Design review of the part built by this model. Coordinates are the model's own, in mm. A direction names the side the tool comes from. Coordinates: 2 decimals unless noted, no trailing zeros. Loops run counter-clockwise (first coordinate to the right, second up) from the corner with the lowest first, then second, coordinate; pieces in that order, holes last. Notation, with made-up numbers: (61, 11.25) - (113, 11.25) arc R15 ccw to (113, 23.25) - close; hole circle Ø11 at (-27, 79). An arc over 180 degrees is marked (long way). One line per question, with ' | ' between items.
from build123d import *

# Parameters (mm, degrees)
PAD_DEPTH       = 3.4
FILLET_R        = 4
SKETCH001_R     = 18
SKETCH001_R_2   = 6.25
PAD001_DEPTH    = 36
SKETCH002_W     = 12
SKETCH002_H     = 42
SKETCH002_R     = 2.65
PAD002_DEPTH    = 48
FILLET002_R     = 2
SKETCH004_W     = 8
SKETCH004_H     = 36.680408
PAD010_DEPTH    = 68
CHAMFER_SIZE    = 20
CHAMFER001_SIZE = 2
SKETCH005_R     = 1.5
POCKET_DEPTH    = 10


with BuildPart() as part:
    # Sketch → Pad (new body)
    with BuildSketch(Plane.XY):
        with BuildLine():
            Line((-65, 0), (-65, -60))
            Line((-65, -60), (65, -60))
            Line((65, -60), (65, 0))
            ThreePointArc((65, 0), (0, 45.409517), (-65, 0))
        make_face()
    extrude(amount=PAD_DEPTH)

    # Fillet
    fillet_edges = [part.edges().sort_by_distance(p)[0] for p in [
        (65, -60, 1.7),
        (-65, -60, 1.7),
    ]]
    fillet(fillet_edges, radius=FILLET_R)

    # Sketch001 (on Face6 of Pad) → Pad001 (join)
    with BuildSketch(Plane.XY.offset(3.4)):
        with Locations((42, -6)):
            Circle(SKETCH001_R)
        with Locations((42, -6)):
            Circle(SKETCH001_R_2, mode=Mode.SUBTRACT)
    pad001 = extrude(amount=PAD001_DEPTH)

    # Mirrored: Pad001 across YZ
    add(pad001.mirror(Plane.YZ))

    # Sketch002 (on Face5 of Mirrored) → Pad002 (join)
    with BuildSketch(Plane.XY.offset(3.4)):
        with Locations((-27.4, -35)):
            Rectangle(SKETCH002_W, SKETCH002_H)
        with Locations((-27.4, -26)):
            Circle(SKETCH002_R, mode=Mode.SUBTRACT)
        with Locations((-27.4, -44)):
            Circle(SKETCH002_R, mode=Mode.SUBTRACT)
    pad002 = extrude(amount=PAD002_DEPTH)

    # Mirrored001: Pad002 across Sketch002 V_Axis
    add(pad002.mirror(Plane(origin=(0, 0, 3.4), x_dir=(0, 0, 1), z_dir=(1, 0, 0))))

    # Fillet002
    fillet002_edges = [part.edges().sort_by_distance(p)[0] for p in [
        (33.4, -14, 45.4),
        (-33.4, -14, 45.4),
    ]]
    fillet(fillet002_edges, radius=FILLET002_R)

    # Sketch004 (on Face6 of Fillet002) → Pad010 (join)
    with BuildSketch(Plane.XY.offset(3.4)):
        with Locations((37.4, -37.659796)):
            Rectangle(SKETCH004_W, SKETCH004_H)
    extrude(amount=PAD010_DEPTH)

    # Chamfer
    chamfer_edges = [part.edges().sort_by_distance(p)[0] for p in [
        (37.4, -56, 71.4),
    ]]
    chamfer(chamfer_edges, length=CHAMFER_SIZE)

    # Chamfer001
    chamfer001_edges = [part.edges().sort_by_distance(p)[0] for p in [
        (33.4, -46, 61.4),
        (33.4, -27.659796, 71.4),
    ]]
    chamfer(chamfer001_edges, length=CHAMFER001_SIZE)

    # Sketch005 (on Face4 of Chamfer001) → Pocket (cut)
    with BuildSketch(Plane.YZ.offset(41.4)):
        with Locations((-32.7462, 64.451439)):
            Circle(SKETCH005_R)
        with Locations((-22.2462, 64.451439)):
            Circle(SKETCH005_R)
    extrude(amount=-POCKET_DEPTH, mode=Mode.SUBTRACT)


solid = part.part
Q1. Take a section at A-A (z = 13). Give the boundary of the cut face in (x, y), plus the area to 3 significant figures.
Returned:
outline: (-33.4, -56) - (-21.4, -56) - (-21.4, -14) - (-25.88, -14) arc R18 ccw (long way) to (-33.4, -21.81) - close; (21.4, -56) - (41.4, -56) - (41.4, -23.99) arc R18 ccw (long way) to (25.88, -14) - (21.4, -14) - close; hole circle Ø12.5 at (-42, -6); hole circle Ø5.3 at (-27.4, -44); hole circle Ø5.3 at (-27.4, -26); hole circle Ø5.3 at (27.4, -44); hole circle Ø5.3 at (27.4, -26); hole circle Ø12.5 at (42, -6) | area: 2,900 mm²
Q2. Take a section at C-C (x = 27.4). Give the boundary of the cut face in (y, z), plus the area to 3 significant figures.
Returned:
outline: (-60, 0) - (39.76, 0) - (39.76, 3.4) - (4.53, 3.4) - (4.53, 39.4) - (-14, 39.4) - (-14, 51.4) - (-23.35, 51.4) - (-23.35, 3.4) - (-28.65, 3.4) - (-28.65, 51.4) - (-41.35, 51.4) - (-41.35, 3.4) - (-46.65, 3.4) - (-46.65, 51.4) - (-56, 51.4) - (-56, 3.4) - (-60, 3.4) - close | area: 2,510 mm²
Q3. To check wall thickness, follow line 1 along Y through (x, z) = (-26.5, 7.5); line 2 along Y through (x, z) = (-42, 27); line 3 along X through (y, z) = (-32, 9.5). State the ranges of each line that lie inside material, in increasing order.
Returned:
line 1: y = -56 to -46.49, -41.51 to -28.49, -23.51 to 3.15 | line 2: y = -24 to -12.25, 0.25 to 12 | line 3: x = -33.4 to -21.4, 21.4 to 41.4
Q4. Take a section at D-D (y = -38). Give the boundary of the cut face in (x, z).
Returned:
outline: (-65, 0) - (65, 0) - (65, 3.4) - (41.4, 3.4) - (41.4, 69.4) - (35.4, 69.4) - (33.4, 66.57) - (33.4, 51.4) - (21.4, 51.4) - (21.4, 3.4) - (-21.4, 3.4) - (-21.4, 51.4) - (-33.4, 51.4) - (-33.4, 3.4) - (-65, 3.4) - close
Q5. For pin 1 (4 mm diameter, centred on x = 28, y = -45, fed in from +Z); pin 2 (11 mm diameter, centred on x = -42.5, y = 1.5, fed in from +Z); pin 3 (13 mm diameter, centred on x = -26.5, z = 19.5, fed in from -Y), all flat-tipped, find the tip position at first contact; note any pin that passes through.
Returned:
pin 1: stops at z = 51.4 | pin 2: stops at z = 39.4 | pin 3: stops at y = -56
Q6. Draft analysis for pull direction X (two halves, no side actions). For faces 1 (the flat face through (28, -35, 51.4)), 2 (the flat face through (24, -14, 32)), 3 (the flat face through (33.4, -18, 45)), state which applies: +X half, -X half, draft (parallel to the pull), parting line (faces both ways), or undercut.
Returned:
face 1: draft | face 2: undercut | face 3: +X half
Q7. Tool access review of faces 4 (the flat face through (33.4, -33, 58)), 5 (the cylindrical face through (-24.95, -27.01, 27.06)), 6 (the flat face through (37, -19.32, 55)), 7 (the flat face through (-27, -56, 27)): name each direction out of +Z, -Z, +X, -X, +Y, -Y from which nothing blocks a thin tool from reaching the whole face with its end or side.
Returned:
face 4: +Z, -X, +Y, -Y | face 5: +Z | face 6: +Z, +X, +Y | face 7: +Z, +X, -X, -Y
Q8. Take a section at B-B (y = -6). Give the boundary of the cut face in (x, z).
Returned:
outline: (-65, 0) - (65, 0) - (65, 3.4) - (60, 3.4) - (60, 39.4) - (48.25, 39.4) - (48.25, 3.4) - (35.75, 3.4) - (35.75, 39.4) - (24, 39.4) - (24, 3.4) - (-24, 3.4) - (-24, 39.4) - (-35.75, 39.4) - (-35.75, 3.4) - (-48.25, 3.4) - (-48.25, 39.4) - (-60, 39.4) - (-60, 3.4) - (-65, 3.4) - close
